For this review, take the finished solid that the model builds, in its own axes (mm). A direction names the side the tool comes from. Coordinates: 2 decimals unless noted, no trailing zeros. Order: outer loops, then holes, each group sorted by start corner. A loop starts at its lowest first (then second) coordinate and runs counter-clockwise, first axis right, second up. Notation, with made-up numbers: (4.25, 1.25) -> (15.25, 1.25) arc R25 cw to (15.25, 38.25) -> close; hole circle Ø4 at (-18.75, 45.25). An arc over 180 degrees is marked (long way). Return JSON: item names as keys, results as strings. Group by question number.
Item 1: Take a section at D-D (z = 0). Write out the cut boundary in (x, y).
Item 2: Take a section at B-B (z = 7.5). Write out the cut boundary in (x, y), then the cut area to 3 significant figures.
Item 3: Insertion check: pin 1 (5.5 mm diameter, centred on x = 5, z = 1, fed in from +Y); pin 2 (11 mm diameter, centred on x = -3.5, y = 60, fed in from +Z); pin 3 (9 mm diameter, centred on x = 1.5, y = 24.5, fed in from +Z). Each pin has a flat end and moves straight along its axis. Give the tip position at first contact, or say it passes through.
Item 4: Take a section at A-A (y = 44.5). Write out the cut boundary in (x, z), then the cut area to 3 significant figures.
Item 5: Machinability: for faces 5 (the flat face through (1, 58, -10)), 6 (the flat face through (12.5, 33, 0)), 7 (the flat face through (-7.75, 28, 1)), 8 (the flat face through (0, 33, 12.5)), which of the approach directions +Z, -Z, +X, -X, +Y, -Y give a long, thin tool a straight path to every point of the face, cutting with its end or side? Answer none if there is none.
Item 6: For line 1 along Z through (x, y) = (-1, 50); line 2 along X through (y, z) = (1, 0); line 3 along Y through (x, z) = (9.5, -1), list the stretches that pass through material, from the lowest coordinate up.
Item 7: Draft analysis for pull direction Z (two halves, no side actions). For faces 1 (the cylindrical face through (16.765, 1.479, -0.806)), 2 (the flat face through (1, 1, 18.3)), 3 (the flat face through (1, 28, 10.25)), 4 (the flat face through (18.3, 1, 0)), state which applies: +Z half, -Z half, draft (parallel to the pull), parting line (faces both ways), or undercut.
Item 8: Take a section at C-C (x = 15.5). Write out the cut boundary in (y, z).
```python
from build123d import *

# Parameters (mm, degrees)
SKETCH1_W           = 25
SKETCH1_H           = 25
BOSS_EXTRUDE1_DEPTH = 63
SKETCH2_W           = 22.5
SKETCH2_H           = 22.5
CUT_EXTRUDE2_DEPTH  = 10
SKETCH4_W           = 25
SKETCH4_H           = 25
SKETCH4_R           = 1.5
BOSS_EXTRUDE2_DEPTH = 3
SKETCH5_W           = 18
SKETCH5_H           = 18
CUT_EXTRUDE3_DEPTH  = 50


with BuildPart() as part:
    # Sketch1 → Boss-Extrude1 (new body)
    with BuildSketch(Plane(origin=(0, 0, 0), x_dir=(1, 0, 0), z_dir=(0, 1, 0))):
        Rectangle(SKETCH1_W, SKETCH1_H)
    extrude(amount=BOSS_EXTRUDE1_DEPTH)

    # Sketch2 → Cut-Extrude2 (cut)
    with BuildSketch(Plane(origin=(0, 63, 0), x_dir=(1, 0, 0), z_dir=(0, 1, 0))):
        with Locations((1.25, -1.25)):
            Rectangle(SKETCH2_W, SKETCH2_H)
    extrude(amount=-CUT_EXTRUDE2_DEPTH, mode=Mode.SUBTRACT)

    # Sketch4 → Boss-Extrude2 (add)
    # profile 1 of 2: a face of its own
    with BuildSketch(Plane.XZ):
        Rectangle(SKETCH4_W, SKETCH4_H)
    # profile 2 of 2: a face of its own
    with BuildSketch(Plane.XZ):
        with BuildLine():
            Line((12.5, 12.5), (12.5, -12.5))
            Line((12.5, -12.5), (18.3, -12.5))
            Line((18.3, -12.5), (18.3, 13.3))
            ThreePointArc((18.3, 13.3), (16.835533906, 16.835533906), (13.3, 18.3))
            Line((13.3, 18.3), (-12.5, 18.3))
            Line((-12.5, 18.3), (-12.5, 12.5))
            Line((-12.5, 12.5), (12.5, 12.5))
        make_face()
        with Locations(Location((15.5, 0, 0), (0, 0, 270))):
            Circle(SKETCH4_R, mode=Mode.SUBTRACT)
        with Locations(Location((0, 15.5, 0), (0, 0, 270))):
            Circle(SKETCH4_R, mode=Mode.SUBTRACT)
    extrude(amount=-BOSS_EXTRUDE2_DEPTH)

    # Sketch5 → Cut-Extrude3 (cut)
    with BuildSketch(Plane(origin=(0, 53, 0), x_dir=(1, 0, 0), z_dir=(0, 1, 0))):
        with Locations((1.25, -1.25)):
            Rectangle(SKETCH5_W, SKETCH5_H)
    extrude(amount=-CUT_EXTRUDE3_DEPTH, mode=Mode.SUBTRACT)


solid = part.part
```
Findings below:
{
 "1": {"outline": "(-12.5, 0) -> (14, 0) -> (14, 3) -> (12.5, 3) -> (12.5, 53) -> (10.25, 53) -> (10.25, 3) -> (-7.75, 3) -> (-7.75, 53) -> (-10, 53) -> (-10, 63) -> (-12.5, 63) -> close; (17, 0) -> (18.3, 0) -> (18.3, 3) -> (17, 3) -> close"},
 "2": {"outline": "(-12.5, 0) -> (18.3, 0) -> (18.3, 3) -> (12.5, 3) -> (12.5, 53) -> (10.25, 53) -> (10.25, 3) -> (-7.75, 3) -> (-7.75, 53) -> (-10, 53) -> (-10, 63) -> (-12.5, 63) -> close", "area": "467 mm2"},
 "3": {"pin 1": "stops at y = 3", "pin 2": "stops at z = -10", "pin 3": "stops at z = 12.5"},
 "4": {"outline": "(-12.5, -12.5) -> (12.5, -12.5) -> (12.5, 12.5) -> (-12.5, 12.5) -> close; hole (-7.75, -7.75) -> (10.25, -7.75) -> (10.25, 10.25) -> (-7.75, 10.25) -> close", "area": "301 mm2"},
 "5": {"face 5": "+Z, +X, +Y", "face 6": "+Z, -Z, +X, +Y", "face 7": "+Y", "face 8": "+Z, +X, -X, +Y"},
 "6": {"line 1": "z = -12.5 to -7.75, 10.25 to 12.5", "line 2": "x = -12.5 to 14, 17 to 18.3", "line 3": "y = 0 to 3"},
 "7": {"face 1": "undercut", "face 2": "+Z half", "face 3": "undercut", "face 4": "draft"},
 "8": {"outline": "(0, -12.5) -> (3, -12.5) -> (3, -1.5) -> (0, -1.5) -> close; (0, 1.5) -> (3, 1.5) -> (3, 17.79) -> (0, 17.79) -> close"}
}
